Autodesk Inventor part; units mm, degrees
ref_plane "YZ Plane" through (0, 0, 0) normal (1, 0, 0) x (0, 1, 0)
ref_plane "XZ Plane" through (0, 0, 0) normal (0, 1, 0) x (-1, 0, 0)
ref_plane "XY Plane" through (0, 0, 0) normal (0, 0, 1) x (1, 0, 0)
sketch "Эскиз1" plane through (0, 0, 0) normal (0, 1, 0) x (-1, 0, 0)
  line L0 (-50, 50) -> (50, 50)
  line L1 (50, 50) -> (50, -50)
  line L2 (50, -50) -> (-50, -50)
  line L3 (-50, -50) -> (-50, 50)
  line L4 (-50, 50) -> (50, -50) construction
  line L5 (50, 50) -> (-50, -50) construction
  line L6 (-35, 35) -> (35, 35)
  line L7 (35, 35) -> (35, -35)
  line L8 (35, -35) -> (-35, -35)
  line L9 (-35, -35) -> (-35, 35)
  line L10 (-35, 35) -> (35, -35) construction
  line L11 (35, 35) -> (-35, -35) construction
  point P0 (0, 0)
  dimension "d0" = 100
  dimension "d1" = 100
  dimension "d2" = 15
  dimension "d3" = 15
extrude "Выдавливание1" add sketch "Эскиз1" along normal blind 50
sketch "Эскиз3" plane through (0, 50, 0) normal (0, 1, 0) x (1, 0, 0)
  line L0 (-35, 35) -> (-35, -35)
  line L1 (-35, 0) -> (-50, 0)
  line L2 (-50, -50) -> (-50, 50)
  line L3 (35, -35) -> (35, 35)
  line L4 (35, 0) -> (50, 0)
  line L5 (50, 50) -> (50, -50)
  line L6 (-35, -20) -> (-50, -20)
  line L7 (-50, -20) -> (-50, 20)
  line L8 (-50, 20) -> (-35, 20)
  line L9 (-35, 20) -> (-35, -20)
  line L10 (-35, -20) -> (-50, 20) construction
  line L11 (-50, -20) -> (-35, 20) construction
  line L12 (50, -20) -> (35, -20)
  line L13 (35, -20) -> (35, 20)
  line L14 (35, 20) -> (50, 20)
  line L15 (50, 20) -> (50, -20)
  line L16 (50, -20) -> (35, 20) construction
  line L17 (35, -20) -> (50, 20) construction
  line L18 (-35, -35) -> (35, -35)
  line L19 (0, -35) -> (0, -50)
  line L20 (50, -50) -> (-50, -50)
  line L21 (35, 35) -> (-35, 35)
  line L22 (0, 35) -> (0, 50)
  line L23 (-50, 50) -> (50, 50)
  line L24 (35, -50) -> (-35, -50)
  line L25 (-35, -50) -> (-35, -35)
  line L26 (-35, -35) -> (35, -35)
  line L27 (35, -35) -> (35, -50)
  line L28 (35, -50) -> (-35, -35) construction
  line L29 (-35, -50) -> (35, -35) construction
  line L30 (35, 50) -> (-35, 50)
  line L31 (-35, 50) -> (-35, 35)
  line L32 (-35, 35) -> (35, 35)
  line L33 (35, 35) -> (35, 50)
  line L34 (35, 50) -> (-35, 35) construction
  line L35 (-35, 50) -> (35, 35) construction
  point P0 (0, 0)
  point P1 (-42.5, 0)
  point P2 (42.5, 0)
  point P3 (0, -42.5)
  point P4 (0, 42.5)
  dimension "d14" = 40
  dimension "d15" = 40
extrude "Выдавливание2" cut sketch "Эскиз3" against normal blind 35 contours L31 L23 L22 L21 | L0 L1 L2 L8 | L22 L23 L33 L21 | L0 L6 L2 L1 | L14 L5 L4 L3 | L18 L19 L20 L25 | L4 L5 L12 L3 | L18 L27 L20 L19
sketch "Эскиз4" plane through (-35, 0, 35) normal (1, 0, 0) x (0, 0, -1)
  line L0 (15, 15) -> (15, 50)
  line L1 (15, 50) -> (0, 50)
  line L2 (0, 50) -> (0, 30)
  line L3 (0, 30) -> (15, 30)
  line L4 (15, 30) -> (15, 50)
  line L5 (85, 50) -> (55, 50)
  line L6 (55, 50) -> (70, 50)
  line L7 (70, 50) -> (70, 30)
  line L8 (70, 30) -> (55, 30)
  line L9 (55, 30) -> (55, 50)
  point P0 (35, 0)
  dimension "d18" = 15
  dimension "d19" = 20
  dimension "d20" = 15
  dimension "d21" = 20
extrude "Выдавливание3" cut sketch "Эскиз4" along normal blind 90.5 and the other way blind 45.25
sketch "Эскиз5" plane through (50, 0, 50) normal (1, 0, 0) x (0, 0, -1)
  circle A0 centre (22.5, 22.5) radius 5.1
  circle A1 centre (77.5, 22.5) radius 5.1
  line L0 (85, 30) -> (70, 30)
  line L1 (70, 30) -> (70, 15)
  line L2 (30, 15) -> (30, 30)
  line L3 (30, 30) -> (15, 30)
  point P0 (50, 0)
  dimension "d26" = 10.2
  dimension "d27" = 10.2
  dimension "d28" = 7.5
  dimension "d29" = 7.5
  dimension "d30" = 7.5
  dimension "d31" = 7.5
extrude "Выдавливание4" cut sketch "Эскиз5" against normal blind 156
sketch "Эскиз6" plane through (0, 50, 0) normal (0, 1, 0) x (1, 0, 0)
  line L0 (-35, 35) -> (-50, 35)
  line L1 (-50, 50) -> (50, 50)
  line L2 (-38.5, 46.5) -> (-46.5, 46.5)
  line L3 (-46.5, 46.5) -> (-46.5, 38.5)
  line L4 (-46.5, 38.5) -> (-38.5, 38.5)
  line L5 (-38.5, 38.5) -> (-38.5, 46.5)
  line L6 (-38.5, 46.5) -> (-46.5, 38.5) construction
  line L7 (-46.5, 46.5) -> (-38.5, 38.5) construction
  line L8 (-50, 50) -> (-50, 35)
  point P0 (0, 0)
  point P1 (-42.5, 42.5)
  dimension "d34" = 8
  dimension "d35" = 8
  dimension "d41" = 7.5
  dimension "d42" = 7.5
extrude "Выдавливание5" add sketch "Эскиз6" along normal blind 20
mirror "Mirror1" about plane through (0, 0, 0) normal (1, 0, 0) of "Выдавливание5"
mirror "Mirror2" about plane through (0, 0, 0) normal (0, 0, 1) of "Выдавливание5", "Mirror1"
properties part number "000.113 - Верх центрального сегмента"
Here's how the part is built. I have some questions about the finished solid (model axes, mm). A direction names the side the tool comes from. Give positions to 0.01 mm unless a question says otherwise; leave off trailing zeros. Write each loop counter-clockwise with the first axis right and the second up, starting at its lowest first coordinate (ties: lowest second). Pieces come first, ordered by that corner, then holes.
(1) Imagine slicing it at A-A, the plane x = 1. Write out the boundary of the cut face in (y, z).
Output values:
outline: (0, -50) - (15, -50) - (15, -35) - (0, -35) - close; (0, 35) - (15, 35) - (15, 50) - (0, 50) - close
(2) On a 3-axis mill with a long thin cutter (end or side, diameter ignored), from which of +Z, -Z, +X, -X, +Y, -Y can I reach the whole of each face in a straight line? I mean faces 1 (the face through (-38.5, 60, -42)), 2 (the face through (-35, 14, 1)), 3 (the face through (0, 7, 35)), 4 (the face through (-43, 23, -20)). Say none if no direction works.
Output values:
face 1: +Z, -Z, +Y
face 2: +Y
face 3: +Y, -Y
face 4: +X, -X, +Y
(3) Imagine slicing it at D-D, the plane z = 27.5. Write out the boundary of the cut face in (x, y), and give its area (3 significant figures).
Output values:
outline: (-50, 0) - (-35, 0) - (-35, 17.4) - (-50, 17.4) - close; (-50, 27.6) - (-35, 27.6) - (-35, 30) - (-50, 30) - close; (35, 0) - (50, 0) - (50, 17.4) - (35, 17.4) - close; (35, 27.6) - (50, 27.6) - (50, 30) - (35, 30) - close
area: 594 mm2
(4) Imagine slicing it at C-C, the plane y = 57.5. Write out the boundary of the cut face in (x, z).
Output values:
outline: (-46.5, -46.5) - (-38.5, -46.5) - (-38.5, -38.5) - (-46.5, -38.5) - close; (-46.5, 38.5) - (-38.5, 38.5) - (-38.5, 46.5) - (-46.5, 46.5) - close; (38.5, -46.5) - (46.5, -46.5) - (46.5, -38.5) - (38.5, -38.5) - close; (38.5, 38.5) - (46.5, 38.5) - (46.5, 46.5) - (38.5, 46.5) - close
(5) Will these pins go through, and if not, where does the flat tip stop? pin 1 (12 mm diameter, centred on x = -41, z = -1, fed in from +Y); pin 2 (7.5 mm diameter, centred on x = 43.5, z = 24.5, fed in from +Y); pin 3 (16.5 mm diameter, centred on x = -44, z = -28, fed in from +Y); pin 4 (13.5 mm diameter, centred on y = 22.5, z = 27.5, fed in from -X).
Output values:
pin 1: stops at y = 15
pin 2: stops at y = 30
pin 3: stops at y = 50
pin 4: stops at x = -50
(6) Thinking about a two-plate mould opening in Z: for faces 5 (the face through (43, 70, 43)), 6 (the face through (-37, 50, 43)), 7 (the face through (42, 60, 46.5)), which applies, pulls with the +Z half, pulls with the -Z half, needs draft (parallel to the pull), parting line crosses it, or undercut?
Output values:
face 5: needs draft
face 6: undercut
face 7: pulls with the +Z half
(7) Imagine slicing it at B-B, the plane z = -15. Write out the boundary of the cut face in (x, y).
Output values:
outline: (-50, 0) - (-35, 0) - (-35, 15) - (-50, 15) - close; (35, 0) - (50, 0) - (50, 15) - (35, 15) - close
(8) If I drill on L1, parallel to Z at x = -40, y = 22; L2, parallel to Y at x = -41.5, z = -27.5; L3, parallel to Z at x = 45, y = 35, over which ranges is the centre line in solid material (lowest first)?
Output values:
L1: z = -50 to -32.58, -22.42 to -20, 20 to 22.42, 32.58 to 50
L2: y = 0 to 17.4, 27.6 to 30
L3: z = -50 to -35, 35 to 50
